```python
from build123d import *

# Parameters (mm, degrees)
SKETCH_1_R          = 1.5
EXTRUDE_1_DEPTH     = 2
SKETCH_2_W          = 2
SKETCH_2_H          = 5
EXTRUDE_2_DEPTH     = 9
SKETCH_3_R          = 1.5
CUT_EXTRUDE_1_DEPTH = 6


with BuildPart() as part:
    # 草图1 → 凸台-拉伸1 (new body)
    with BuildSketch(Plane(origin=(0, 0, 0), x_dir=(0, 0, -1), z_dir=(1, 0, 0))):
        Polygon((-11, 0), (-11, 2.5), (0, 2.5), (0, 0), (0, -2.5), (-11, -2.5), align=None)
        with Locations((-8, 0)):
            Circle(SKETCH_1_R, mode=Mode.SUBTRACT)
    extrude(amount=EXTRUDE_1_DEPTH)

    # 草图2 → 凸台-拉伸2 (add)
    with BuildSketch(Plane(origin=(2, 0, 0), x_dir=(0, 0, -1), z_dir=(1, 0, 0))):
        with Locations((-1, 0)):
            Rectangle(SKETCH_2_W, SKETCH_2_H)
    extrude(amount=EXTRUDE_2_DEPTH)

    # 草图3 → 切除-拉伸1 (cut)
    with BuildSketch(Plane.XY.offset(2)):
        with Locations((8, 0)):
            Circle(SKETCH_3_R)
    extrude(amount=-CUT_EXTRUDE_1_DEPTH, mode=Mode.SUBTRACT)


solid = part.part
```
Build history of the part. All positions in model axes, mm. A direction names the side the tool comes from. Round coordinates to 2 decimals unless told otherwise and drop trailing zeros. Loops run counter-clockwise (first coordinate to the right, second up) from the corner with the lowest first, then second, coordinate; pieces in that order, holes last. Notation, with made-up numbers: M -20.75,10.5 L 22.25,10.5 A16 ccw 22.25,22.5 Z; hole C 85.25,57 d9. An arc over 180 degrees is marked long. Answer as CSV lines item,"result".
1. Cut at C-C on y = 0. Write the cut outline in (x, z), then the cut area to 3 significant figures.
Resolved:
outline,"M 0,0 L 6.5,0 L 6.5,2 L 2,2 L 2,6.5 L 0,6.5 Z; M 0,9.5 L 2,9.5 L 2,11 L 0,11 Z; M 9.5,0 L 11,0 L 11,2 L 9.5,2 Z"
area,"28.0 mm²"
2. Cut at A-A on z = 8. Write the cut outline in (x, y).
Resolved:
outline,"M 0,-2.5 L 2,-2.5 L 2,-1.5 L 0,-1.5 Z; M 0,1.5 L 2,1.5 L 2,2.5 L 0,2.5 Z"
3. Cut at B-B on x = 8. Write the cut outline in (y, z), then the cut area to 3 significant figures.
Resolved:
outline,"M -2.5,0 L -1.5,0 L -1.5,2 L -2.5,2 Z; M 1.5,0 L 2.5,0 L 2.5,2 L 1.5,2 Z"
area,"4.00 mm²"
4. Wall check: probe 1 along Z at (x, y) = (1.5, 0.1); probe 2 along Y at (x, z) = (0.45, 8); probe 3 along X at (y, z) = (0.5, 2.75). Give the ranges that are in metal, low to high. Write a range as [from, to].
Resolved:
probe 1,"z = [0, 6.5], [9.5, 11]"
probe 2,"y = [-2.5, -1.5], [1.5, 2.5]"
probe 3,"x = [0, 2]"
5. Two-plate mould, pull along X, no slides. Class faces 1 (the flat face through (2, 0, 6)), 2 (the flat face through (0, 0, 5)), 3 (the flat face through (1, 0, 11)), 4 (the cylindrical face through (6.5, 0.07, 1.01)): released by +X, released by -X, zero draft, split by the parting line, or undercut.
Resolved:
face 1,"released by +X"
face 2,"released by -X"
face 3,"zero draft"
face 4,"undercut"
6. Cut at D-D on z = 1. Write the cut outline in (x, y).
Resolved:
outline,"M 0,-2.5 L 11,-2.5 L 11,2.5 L 0,2.5 Z; hole C 8,0 d3"
7. 3-axis set-ups, long thin cutter, end or side, ignore diameter. For faces 5 (the flat face through (5, 0, 0)), 6 (the flat face through (6, 0, 2)): which of +Z, -Z, +X, -X, +Y, -Y reach the whole face in a straight line?
Resolved:
face 5,"-Z, +X, -X, +Y, -Y"
face 6,"+Z, +X, +Y, -Y"
8. Flat gauge pins, fed straight in: P1, Ø2.5, axis at x = 4.5, y = -1, coming from the +Z side; P2, Ø1.5, axis at x = 7.5, y = -1.5, coming from the -Z side; P3, Ø2.5, axis at y = -1, z = 6, coming from the +X side. Where does each tip first touch, or does it go through?
Resolved:
P1,"stops at z = 2"
P2,"stops at z = 0"
P3,"stops at x = 2"
